Autodesk Inventor part; units mm, degrees
ref_plane "IDS_WORKPLANE{1}" through (-4.6, 0, 0) normal (1, 0, 0) x (0, 0, -1)
ref_plane "Work Plane2" through (69.85, 0, 0) normal (0, 0, -1) x (1, 0, 0)
ref_plane "YZ Plane" through (0, 0, 0) normal (1, 0, 0) x (0, 1, 0)
sketch "Sketch1" plane through (0, 0, 0) normal (0, 0, 1) x (1, 0, 0)
  line L0 (-0.59, 0) -> (13, 0)
  line L1 (13, 0) -> (13, 3)
  line L2 (13, 3) -> (0, 3)
  line L3 (0, 3) -> (0, 6)
  line L4 (-8.7003, 0) -> (16.6167, 0)
  line L5 (0, -1.2172) -> (0, 7.3031)
  line L6 (-4.6, 2.3998) -> (-5.0836, 2.3998) construction
  line L7 (-4.6, 0) -> (-0.59, 0)
  line L8 (0, 0) -> (-0.59, 0)
  line L9 (-4.6, 0) -> (-4.6, 6)
  arc A0 (-2.8922, 6) -> (-4.6, 2.3998) centre (5.1078, 0) ccw
  line L10 (-4.6, 6) -> (0, 6)
  dimension "d0" = 13
  dimension "d1" = 6
  dimension "d2" = 12
  dimension "d4" = 4.7996
  dimension "d13" = 4.6
  dimension "d14" = 4.01
  dimension "d46" = 10
  dimension "d47" = 0
revolve "Body" add sketch "Sketch1" angle 360 about axis through (-0.59, 0, 0) along (1, 0, 0) contours L4 L9 A0 L10 L3 L5 L0 | L5 L2 L1 L0
ref_plane "IDS_WORKPLANE{1}" through (-4.6, 0, 0) normal (1, 0, 0) x (0, 0, -1)
sketch "Sketch2" plane through (-4.6, 0, 0) normal (1, 0, 0) x (0, 0, -1)
  line L0 (0, -8.4) -> (0, 8.4)
  line L1 (8.4, 0) -> (-8.4, 0)
  line L2 (-1.289, 1.289) -> (1.289, 1.289)
  line L3 (1.289, 1.289) -> (1.289, -1.289)
  line L4 (1.289, -1.289) -> (-1.289, -1.289)
  line L5 (-1.289, -1.289) -> (-1.289, 1.289)
  line L6 (0, 1.289) -> (0, -1.289) construction
  line L7 (-1.289, 0) -> (1.289, 0) construction
  dimension "d7" = 2.578
  dimension "d9" = 2.578
extrude "Extrusion" cut sketch "Sketch2" along normal blind 4.01
fillet "Fillet1" radius 1.289 4 edges at (-0.59, 0, -1.289) (-0.59, -1.289, 0) (-0.59, 0, 1.289) (-0.59, 1.289, 0)
chamfer "Chamfer1" distance 0.401 angle 45 4 edges at (-4.6, 1.289, 0) (-4.6, 0, -1.289) (-4.6, -1.289, 0) (-4.6, 0, 1.289)
thread "Thread"
chamfer "Chamfer2" distance 0.875 distance2 0.6135 1 edges at (13, -3, 0) measured on face at (13, -1.1424, 0.935)
ref_plane "Work Plane2" through (69.85, 0, 0) normal (0, 0, -1) x (1, 0, 0)
fillet "Fillet2" radius 0.3 1 edges at (0, -3, 0)
equation "\"d0\" = NLG"
equation "\"d1\" = GD"
equation "\"d2\" = KOD"
equation "\"d4\" = 1.42 * KOM"
equation "\"d13\" = KOH"
equation "\"d14\" = STI"
equation "\"d46\" = KR"
equation "\"d7\" = KOM - 0.2 * STI"
equation "\"d9\" = KOM - 0.2 * STI"
equation "\"d48\" = STI"
equation "\"d50\" = -0.1 * STI + 0.5 * KOM"
equation "\"d51\" = 0.1 * STI"
equation "\"d18\" = GEL"
equation "\"d20\" = -0.5 * SPD + 0.5 * GD"
equation "\"d21\" = GUL"
equation "\"d44\" = R"
equation "\"GD\" = 6"
equation "\"NLG\" = 13"
equation "\"GEL\" = 12"
equation "\"KOD\" = 12"
equation "\"KOH\" = 4.6"
equation "\"SPD\" = 4.25"
equation "\"KR\" = 10"
equation "\"RR\" = 2"
equation "\"GUL\" = 0.61345 * PTC"
equation "\"KEWI\" = 0"
equation "\"SDM\" = 3.38"
equation "\"STI\" = 4.01"
equation "\"d6\" = -KOH"
equation "\"R\" = 0.3"
equation "\"KOM\" = 3.38"
equation "\"PTC\" = 1"
properties part number "ANSI B18.6.7M - M6x1 x 13, SRPHMSTIM" material "Steel, Mild"
Can you work these out from the model? Positions are in its coordinate system, mm. A direction names the side the tool comes from. Give positions to 0.01 mm unless a question says otherwise; leave off trailing zeros. Loops run counter-clockwise (first coordinate to the right, second up) from the corner with the lowest first, then second, coordinate; pieces in that order, holes last. Notation, with made-up numbers: M 27,18 L 55,18 A22 cw 55,33 Z; hole C 78,6.5 d5. An arc over 180 degrees is marked long. Use CSV: the item, a comma, the result in double quotes. Start each with the question number.
1. If we mould it in two halves opening along Z, with no side actions, what happens to faces 4 (the face through (-1.13, 1.05, 0.02)), 5 (the face through (-4.6, 0, -2)), 6 (the face through (-1, -6, 0))? For each: released by +Z, released by -Z, zero draft, split by the parting line, or undercut.
2. For P1, Ø1.9, axis at x = -3.5, z = -0.5, coming from the -Y side; P2, Ø2, axis at x = 9.5, z = -1, coming from the +Y side; P3, Ø3, axis at y = -4, z = 0, coming from the +X side; P4, Ø1, axis at x = -1.5, z = -4, coming from the -Y side, each with a flat end and sliding along its axis, tell me the tip position at first contact or that it passes through.
3. On a 3-axis mill with a long thin cutter (end or side, diameter ignored), from which of +Z, -Z, +X, -X, +Y, -Y can I reach the whole of each face in a straight line? I mean faces 1 (the face through (6, -3, 0)), 2 (the face through (-3, 1.289, 0)), 3 (the face through (13, 0, 0)). Say none if no direction works.
4. If I drill on L1, parallel to Y at x = -2.75, z = 0.75; L2, parallel to Y at x = -0.5, z = 0.25; L3, parallel to Y at x = -3, z = -0.25, over which ranges is the centre line in solid material (lowest first)?
5. Imagine slicing it at A-A, the plane x = 11.25. Write out the boundary of the cut face in (y, z).
Response values:
1,face 4,"undercut"
1,face 5,"zero draft"
1,face 6,"split by the parting line"
2,P1,"y = -6"
2,P2,"y = 3"
2,P3,"x = 12.74"
2,P4,"y = -4.87"
3,face 1,"+X"
3,face 2,"-X"
3,face 3,"+Z, -Z, +X, +Y, -Y"
4,L1,"-5.95 to -1.29, 1.29 to 5.95"
4,L2,"-5.99 to 5.99"
4,L3,"-5.85 to -1.29, 1.29 to 5.85"
5,outline,"C 0,0 d6"
